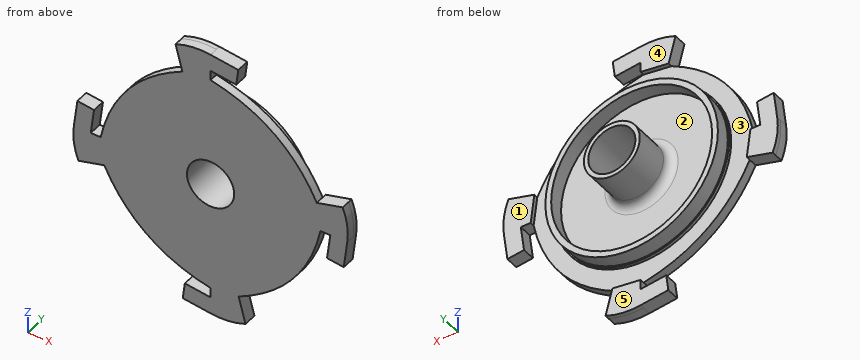
from build123d import *

# Parameters (mm, degrees)
BOSS_EXTRUDE1_DEPTH = 3
BOSS_EXTRUDE2_START = 3
BOSS_EXTRUDE2_DEPTH = 1.5
SKETCH2_R           = 30.3
SKETCH2_R_2         = 29.8
SKETCH2_R_3         = 27.8
BOSS_EXTRUDE3_DEPTH = 1
SKETCH3_R           = 29.8
SKETCH3_R_2         = 27.8
BOSS_EXTRUDE4_DEPTH = 5
SKETCH4_R           = 9.65
SKETCH4_R_2         = 8.15
BOSS_EXTRUDE5_DEPTH = 15
FILLET1_R           = 3
SKETCH5_R           = 8.15
CUT_EXTRUDE1_DEPTH  = 19


with BuildPart() as part:
    # Sketch1 → Boss-Extrude1 (new body)
    with BuildSketch(Plane(origin=(0, 0, 0), x_dir=(1, 0, 0), z_dir=(0, 1, 0))):
        with BuildLine():
            add(Edge.make_bspline(
                [(-9.71796746, -36.684650856), (-32.908122366, -25.325665089), (-37.95, 0)],
                knots=[0, 0, 0, 1, 1, 1], degree=2))
            Line((-37.95, 0), (-36.684650856, 9.71796746))
            add(Edge.make_bspline(
                [(-36.684650856, 9.71796746), (-25.325665089, 32.908122366), (0, 37.95)],
                knots=[0, 0, 0, 1, 1, 1], degree=2))
            Line((0, 37.95), (9.71796746, 36.684650856))
            add(Edge.make_bspline(
                [(9.71796746, 36.684650856), (32.908122366, 25.325665089), (37.95, 0)],
                knots=[0, 0, 0, 1, 1, 1], degree=2))
            Line((37.95, 0), (36.684650856, -9.71796746))
            add(Edge.make_bspline(
                [(36.684650856, -9.71796746), (25.325665089, -32.908122366), (0, -37.95)],
                knots=[0, 0, 0, 1, 1, 1], degree=2))
            Line((0, -37.95), (-9.71796746, -36.684650856))
        make_face()
        with BuildLine():
            Line((-36.684650856, 9.71796746), (-45.626232422, 12.086642005))
            add(Edge.make_bspline(
                [(-45.626232422, 12.086642005), (-47.200054133, 8.194360075), (-47.724535059, 4.165503049), (-47.2, 0)],
                knots=[0, 0, 0, 0, 1, 1, 1, 1], degree=3))
            Line((-47.2, 0), (-45.991859888, -9.594232511))
            Line((-45.991859888, -9.594232511), (-40.237304711, -8.869598317))
            Line((-40.237304711, -8.869598317), (-41.354196291, 0))
            Line((-41.354196291, 0), (-37.95, 0))
            Line((-37.95, 0), (-36.684650856, 9.71796746))
        make_face()
        with BuildLine():
            Line((-9.71796746, -36.684650856), (-12.086642005, -45.626232422))
            add(Edge.make_bspline(
                [(-12.086642005, -45.626232422), (-8.194360105, -47.200054362), (-4.165503019, -47.72453483), (0, -47.2)],
                knots=[0, 0, 0, 0, 1, 1, 1, 1], degree=3))
            Line((0, -47.2), (9.594232575, -45.991860399))
            Line((9.594232575, -45.991860399), (8.869598688, -40.237305183))
            Line((8.869598688, -40.237305183), (0, -41.35419633))
            Line((0, -41.35419633), (0, -37.95))
            Line((0, -37.95), (-9.71796746, -36.684650856))
        make_face()
        with BuildLine():
            add(Edge.make_bspline(
                [(47.2, 0), (47.724535051, -4.165503048), (47.200054142, -8.194360076), (45.626232422, -12.086642005)],
                knots=[0, 0, 0, 0, 1, 1, 1, 1], degree=3))
            Line((45.626232422, -12.086642005), (36.684650856, -9.71796746))
            Line((36.684650856, -9.71796746), (37.95, 0))
            Line((37.95, 0), (41.354196292, 0))
            Line((41.354196292, 0), (40.237304729, 8.869598332))
            Line((40.237304729, 8.869598332), (45.991859908, 9.594232513))
            Line((45.991859908, 9.594232513), (47.2, 0))
        make_face()
        with BuildLine():
            Line((9.71796746, 36.684650856), (12.086642005, 45.626232422))
            add(Edge.make_bspline(
                [(12.086642005, 45.626232422), (8.194360088, 47.200054234), (4.165503036, 47.724534958), (0, 47.2)],
                knots=[0, 0, 0, 0, 1, 1, 1, 1], degree=3))
            Line((0, 47.2), (-9.594232539, 45.991860113))
            Line((-9.594232539, 45.991860113), (-8.869598481, 40.237304919))
            Line((-8.869598481, 40.237304919), (0, 41.354196308))
            Line((0, 41.354196308), (0, 37.95))
            Line((0, 37.95), (9.71796746, 36.684650856))
        make_face()
    extrude(amount=BOSS_EXTRUDE1_DEPTH)

    # Sketch1<3> → Boss-Extrude2 (add)
    with BuildSketch(Plane(origin=(0, 0, 0), x_dir=(1, 0, 0), z_dir=(0, 1, 0)).offset(BOSS_EXTRUDE2_START)):
        with BuildLine():
            Line((-9.71796746, -36.684650856), (-12.086642005, -45.626232422))
            add(Edge.make_bspline(
                [(-12.086642005, -45.626232422), (-8.194360105, -47.200054362), (-4.165503019, -47.72453483), (0, -47.2)],
                knots=[0, 0, 0, 0, 1, 1, 1, 1], degree=3))
            Line((0, -47.2), (9.594232575, -45.991860399))
            Line((9.594232575, -45.991860399), (8.869598688, -40.237305183))
            Line((8.869598688, -40.237305183), (0, -41.35419633))
            Line((0, -41.35419633), (0, -37.95))
            Line((0, -37.95), (-9.71796746, -36.684650856))
        make_face()
        with BuildLine():
            add(Edge.make_bspline(
                [(47.2, 0), (47.724535051, -4.165503048), (47.200054142, -8.194360076), (45.626232422, -12.086642005)],
                knots=[0, 0, 0, 0, 1, 1, 1, 1], degree=3))
            Line((45.626232422, -12.086642005), (36.684650856, -9.71796746))
            Line((36.684650856, -9.71796746), (37.95, 0))
            Line((37.95, 0), (41.354196292, 0))
            Line((41.354196292, 0), (40.237304729, 8.869598332))
            Line((40.237304729, 8.869598332), (45.991859908, 9.594232513))
            Line((45.991859908, 9.594232513), (47.2, 0))
        make_face()
        with BuildLine():
            Line((9.71796746, 36.684650856), (12.086642005, 45.626232422))
            add(Edge.make_bspline(
                [(12.086642005, 45.626232422), (8.194360088, 47.200054234), (4.165503036, 47.724534958), (0, 47.2)],
                knots=[0, 0, 0, 0, 1, 1, 1, 1], degree=3))
            Line((0, 47.2), (-9.594232539, 45.991860113))
            Line((-9.594232539, 45.991860113), (-8.869598481, 40.237304919))
            Line((-8.869598481, 40.237304919), (0, 41.354196308))
            Line((0, 41.354196308), (0, 37.95))
            Line((0, 37.95), (9.71796746, 36.684650856))
        make_face()
        with BuildLine():
            Line((-36.684650856, 9.71796746), (-45.626232422, 12.086642005))
            add(Edge.make_bspline(
                [(-45.626232422, 12.086642005), (-47.200054133, 8.194360075), (-47.724535059, 4.165503049), (-47.2, 0)],
                knots=[0, 0, 0, 0, 1, 1, 1, 1], degree=3))
            Line((-47.2, 0), (-45.991859888, -9.594232511))
            Line((-45.991859888, -9.594232511), (-40.237304711, -8.869598317))
            Line((-40.237304711, -8.869598317), (-41.354196291, 0))
            Line((-41.354196291, 0), (-37.95, 0))
            Line((-37.95, 0), (-36.684650856, 9.71796746))
        make_face()
    extrude(amount=BOSS_EXTRUDE2_DEPTH)

    # Sketch2 → Boss-Extrude3 (add)
    with BuildSketch(Plane(origin=(0, 3, 0), x_dir=(1, 0, 0), z_dir=(0, 1, 0))):
        Circle(SKETCH2_R)
        Circle(SKETCH2_R_2, mode=Mode.SUBTRACT)
        Circle(SKETCH2_R_2)
        Circle(SKETCH2_R_3, mode=Mode.SUBTRACT)
        Circle(SKETCH2_R_3)
    extrude(amount=BOSS_EXTRUDE3_DEPTH)

    # Sketch3 → Boss-Extrude4 (add)
    with BuildSketch(Plane(origin=(0, 4, 0), x_dir=(1, 0, 0), z_dir=(0, 1, 0))):
        Circle(SKETCH3_R)
        Circle(SKETCH3_R_2, mode=Mode.SUBTRACT)
    extrude(amount=BOSS_EXTRUDE4_DEPTH)

    # Sketch4 → Boss-Extrude5 (add)
    with BuildSketch(Plane(origin=(0, 4, 0), x_dir=(1, 0, 0), z_dir=(0, 1, 0))):
        Circle(SKETCH4_R)
        Circle(SKETCH4_R_2, mode=Mode.SUBTRACT)
    extrude(amount=BOSS_EXTRUDE5_DEPTH)

    # Fillet1
    fillet1_edges = [part.edges().sort_by_distance(p)[0] for p in [
        (-9.65, 4, 0),
    ]]
    fillet(fillet1_edges, radius=FILLET1_R)

    # Sketch5 → Cut-Extrude1 (cut)
    with BuildSketch(Plane.XZ):
        Circle(SKETCH5_R)
    extrude(amount=-CUT_EXTRUDE1_DEPTH, mode=Mode.SUBTRACT)


solid = part.part
Could you check a few things on this model? Use its own coordinates, in mm. Face numbers are marked on the shaded views. A direction names the side the tool comes from. Give positions to 0.01 mm unless a question says otherwise; leave off trailing zeros. Write each loop counter-clockwise with the first axis right and the second up, starting at its lowest first coordinate (ties: lowest second). Pieces come first, ordered by that corner, then holes. Notation, with made-up numbers: (36.25, 45.25) -> (45.25, 45.25) arc R30 ccw to (45.25, 67.25) -> close; hole circle Ø9 at (8.25, 2). An arc over 180 degrees is marked (long way). Answer as a JSON object with one key per item and string values.
Q1. Please list where these lines run through material, in increasing order: L1, parallel to Z at x = 0, y = 7.5; L2, parallel to X at y = 13, z = 0.
Taken from the geometry:
{"L1": "z = -29.8 to -27.8, -9.65 to -8.15, 8.15 to 9.65, 27.8 to 29.8", "L2": "x = -9.65 to -8.15, 8.15 to 9.65"}
Q2. Suppose I cut it at B-B on x = -4. Count the separate pieces of the cut face and the enclosed holes in it, then the cut area to 3 significant figures.
Taken from the geometry:
{"separate pieces": "3", "enclosed holes": "0", "area": "373 mm²"}
Q3. Suppose I cut it at A-A on y = 13. Write out the boundary of the cut face in (x, z), then the cut area to 3 significant figures.
Taken from the geometry:
{"outline": "circle Ø19.3 at (0, 0); hole circle Ø16.3 at (0, 0)", "area": "83.9 mm²"}
Q4. We'd pull the mould along X, two halves only. Please class the marked faces 1 and 2: released by +X, released by -X, zero draft, split by the parting line, or undercut.
Taken from the geometry:
{"face 1": "zero draft", "face 2": "undercut"}
Q5. Will these pins go through, and if not, where does the flat tip stop? pin 1 Ø3.5 at (x, y) = (40, 1.5) entering from -Z; pin 2 Ø3 at (x, z) = (-3.5, 43) entering from +Y; pin 3 Ø3.5 at (y, z) = (2.5, 39.5) entering from +X.
Taken from the geometry:
{"pin 1": "stops at z = -9.06", "pin 2": "stops at y = 4.5", "pin 3": "stops at x = 9"}
Q6. Which directions (+Z, -Z, +X, -X, +Y, -Y) give clear straight access to the entire face, cutting with the end or side of a thin tool? Please do the marked faces 3, 4 and 5.
Taken from the geometry:
{"face 3": "+Y", "face 4": "+Z, +X, -X, +Y", "face 5": "-Z, +X, -X, +Y"}
